Geometry check sheet. Reference: the model listing, model coordinates, mm. Give positions to 0.01 mm unless a question says otherwise; leave off trailing zeros. Write each loop counter-clockwise with the first axis right and the second up, starting at its lowest first coordinate (ties: lowest second). Pieces come first, ordered by that corner, then holes.
(1) Cross-section at A-A (x = -10). Record the boundary of the cut face in (y, z) (3 decimals).
(2) Thickness scan on line 1 along X through (y, z) = (14, 10); line 2 along Z through (x, y) = (10.75, 1.25). Record the ranges inside material, lowest first.
(3) Cross-section at C-C (y = 12). Record the boundary of the cut face in (x, z), and give its area (3 significant figures).
(4) Cross-section at B-B (z = 10). Record the boundary of the cut face in (x, y) (3 decimals), and give its area (3 significant figures).
(5) Mould release check, pull along X, two halves, no side actions. Record for faces 1 (the cylindrical face through (12.6, 9.13, 12.64)), 2 (the flat face through (-13.5, 9, 0)), 3 (the cylindrical face through (10.97, 8.87, 11.27)): +X half, -X half, draft (parallel to the pull), parting line (faces both ways), or undercut.
```python
from build123d import *

# Parameters (mm, degrees)
SKETCH1_W                     = 27
SKETCH1_H                     = 27
BOSS_EXTRUDE1_DEPTH           = 18
M3_CLEARANCE_HOLE1_AT_2_COUNT = 2
M3_CLEARANCE_HOLE1_AT_2_PITCH = 20
M3_CLEARANCE_HOLE1_AT_3_COUNT = 2
M3_CLEARANCE_HOLE1_AT_3_PITCH = 28.284271247
M3_CLEARANCE_HOLE1_AT_4_COUNT = 2
M3_CLEARANCE_HOLE1_AT_4_PITCH = 20
FILLET1_R                     = 3


with BuildPart() as part:
    # Sketch1 → Boss-Extrude1 (new body)
    with BuildSketch(Plane(origin=(0, 0, 0), x_dir=(1, 0, 0), z_dir=(0, 1, 0))):
        Rectangle(SKETCH1_W, SKETCH1_H)
    extrude(amount=BOSS_EXTRUDE1_DEPTH)

    # Sketch4 → M3 Clearance Hole1 (revolve, cut)
    with BuildSketch(Plane(origin=(10, 0, -10), x_dir=(0, 0, -1), z_dir=(1, 0, 0))):
        Polygon((0, 0), (0, 18), (1.625, 18), (1.6, 17.975), (1.6, 0.025), (1.625, 0), align=None)
    m3_clearance_hole1 = revolve(axis=Axis((10, -6.35, -10), (0, 1, 0)), mode=Mode.SUBTRACT)

    # M3 Clearance Hole1 at 2: M3 Clearance Hole1 ×2
    with Locations(*[(-i * M3_CLEARANCE_HOLE1_AT_2_PITCH, 0, 0) for i in range(1, M3_CLEARANCE_HOLE1_AT_2_COUNT)]):
        add(m3_clearance_hole1, mode=Mode.SUBTRACT)

    # M3 Clearance Hole1 at 3: M3 Clearance Hole1 ×2
    with Locations(*[Vector(-0.7071067811865476, 0, 0.7071067811865475) * (i * M3_CLEARANCE_HOLE1_AT_3_PITCH) for i in range(1, M3_CLEARANCE_HOLE1_AT_3_COUNT)]):
        add(m3_clearance_hole1, mode=Mode.SUBTRACT)

    # M3 Clearance Hole1 at 4: M3 Clearance Hole1 ×2
    with Locations(*[(0, 0, i * M3_CLEARANCE_HOLE1_AT_4_PITCH) for i in range(1, M3_CLEARANCE_HOLE1_AT_4_COUNT)]):
        add(m3_clearance_hole1, mode=Mode.SUBTRACT)

    # Fillet1
    fillet1_edges = [part.edges().sort_by_distance(p)[0] for p in [
        (-13.5, 9, -13.5),
        (13.5, 9, -13.5),
        (13.5, 9, 13.5),
        (-13.5, 9, 13.5),
    ]]
    fillet(fillet1_edges, radius=FILLET1_R)


solid = part.part
```
Reply:
1. outline: (0, -13.5) - (18, -13.5) - (18, -11.625) - (17.975, -11.6) - (0.025, -11.6) - (0, -11.625) - close; (0, -8.375) - (0.025, -8.4) - (17.975, -8.4) - (18, -8.375) - (18, 8.375) - (17.975, 8.4) - (0.025, 8.4) - (0, 8.375) - close; (0, 11.625) - (0.025, 11.6) - (17.975, 11.6) - (18, 11.625) - (18, 13.5) - (0, 13.5) - close
2. line 1: x = -13.5 to -11.6, -8.4 to 8.4, 11.6 to 13.5
2. line 2: z = -13.49 to -11.41, -8.59 to 8.59, 11.41 to 13.49
3. outline: (-13.5, -10.5) arc R3 ccw to (-10.5, -13.5) - (10.5, -13.5) arc R3 ccw to (13.5, -10.5) - (13.5, 10.5) arc R3 ccw to (10.5, 13.5) - (-10.5, 13.5) arc R3 ccw to (-13.5, 10.5) - close; hole circle Ø3.2 at (-10, -10); hole circle Ø3.2 at (-10, 10); hole circle Ø3.2 at (10, -10); hole circle Ø3.2 at (10, 10)
3. area: 689 mm2
4. outline: (-13.5, 0) - (-11.625, 0) - (-11.6, 0.025) - (-11.6, 17.975) - (-11.625, 18) - (-13.5, 18) - close; (-8.4, 0.025) - (-8.375, 0) - (8.375, 0) - (8.4, 0.025) - (8.4, 17.975) - (8.375, 18) - (-8.375, 18) - (-8.4, 17.975) - close; (11.6, 0.025) - (11.625, 0) - (13.5, 0) - (13.5, 18) - (11.625, 18) - (11.6, 17.975) - close
4. area: 371 mm2
5. face 1: +X half
5. face 2: -X half
5. face 3: undercut
